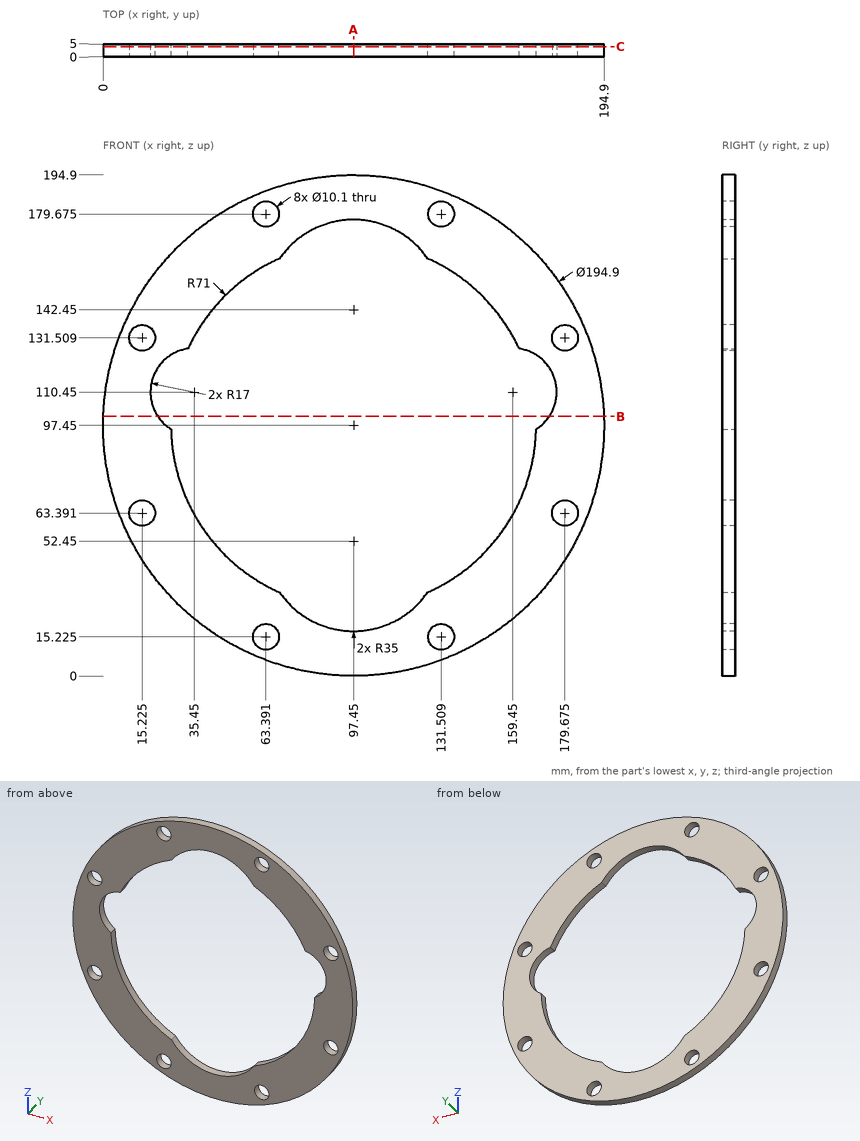
Part print with two shaded views. Sizes in mm from the minimum x, y, z corner. Round coordinates to 2 decimals unless told otherwise and drop trailing zeros. Order: outer loops, then holes, each group sorted by start corner. A loop starts at its lowest first (then second) coordinate and runs counter-clockwise, first axis right, second up. Notation, with made-up numbers: (-8.5, 32) - (18.5, 32) arc R5 cw to (18.5, 37) - close; hole circle Ø6 at (-39.5, 87.5). An arc over 180 degrees is marked (long way). Answer in a Markdown table with one row per item. Add a question column.
(1) Band-saw the part on C-C on y = 4. Count the separate pieces of the cut face and the enclosed holes in it, and give its area (3 significant figures).
(2) Drop flat-ended pins along their axis: pin 1 Ø8 at (x, z) = (15.22, 63.39) entering from +Y; pin 2 Ø3 at (y, z) = (4, 147.5) entering from +X (1 decimal). Give the stop position or say it passes through.
(3) Band-saw the part on B-B on z = 101. List the corners of the cut face in (x, y) (1 decimal).
(4) Probe L1, parallel to Z at x = 67, y = 2; L2, parallel to X at y = 3.5, z = 133.5 (1 decimal); L3, parallel to X at y = 1.4, z = 131. List the from-to ranges inside material, lowest first. Write a range as [from, to].
(5) Band-saw the part on A-A on x = 97.45. List the corners of the cut face in (y, z).
Data:
| question | item | result |
|---|---|---|
| 1 | separate pieces | 1 |
| 1 | enclosed holes | 9 |
| 1 | area | 12,200 mm^2 |
| 2 | pin 1 | passes through |
| 2 | pin 2 | stops at x = 181.9 |
| 3 | outline | (0.1, 0) - (21.3, 0) - (21.3, 5) - (0.1, 5) - close; (173.6, 0) - (194.8, 0) - (194.8, 5) - (173.6, 5) - close |
| 4 | L1 | z = [4.88, 11.69], [18.76, 33.31], [161.59, 176.14], [183.21, 190.02] |
| 4 | L2 | x = [6.9, 10.6], [19.9, 36.3], [158.6, 175], [184.3, 188] |
| 4 | L3 | x = [5.96, 10.2], [20.25, 34.88], [160.02, 174.65], [184.7, 188.94] |
| 5 | outline | (0, 0) - (5, 0) - (5, 17.45) - (0, 17.45) - close; (0, 177.45) - (5, 177.45) - (5, 194.9) - (0, 194.9) - close |
